Autodesk Inventor part; units mm, degrees
ref_plane "YZ Plane" through (0, 0, 0) normal (1, 0, 0) x (0, 1, 0)
ref_plane "XZ Plane" through (0, 0, 0) normal (0, 1, 0) x (-1, 0, 0)
ref_plane "XY Plane" through (0, 0, 0) normal (0, 0, 1) x (1, 0, 0)
sketch "スケッチ1" plane through (0, 0, 0) normal (1, 0, 0) x (0, 1, 0)
  line L0 (-670, 192.9198) -> (-670, 500)
  line L1 (-670, 500) -> (-350, 650)
  line L2 (-350, 650) -> (-90, 650)
  line L3 (0, 250) -> (0, 0)
  line L4 (-124.5856, 512.0252) -> (-145.1979, 512.0252)
  line L5 (-145.1979, 512.0252) -> (0, 250)
  line L6 (-90, 650) -> (-124.5856, 512.0252)
  line L7 (-249.1712, 52.2397) -> (-510, 192.9198)
  line L8 (-510, 192.9198) -> (-670, 192.9198)
  line L9 (0, 0) -> (-249.1712, 52.2397)
  dimension "d2" = 150
  dimension "d3" = 320
  dimension "d4" = 250
  dimension "d5" = 670
  dimension "d79" = 260
extrude "押し出し1" add sketch "スケッチ1" along normal blind 5
sketch "スケッチ8" plane through (5, 0, 0) normal (1, 0, 0) x (0, 0, -1)
  circle A0 centre (-570, -250) radius 7.5
  circle A1 centre (-288.2903, -224.7089) radius 7.5
  line L0 (0, 0) -> (-250, 0)
  line L1 (-570, -250) -> (-290.3837, -264.6541)
  line L2 (-290.3837, -264.6541) -> (-288.2903, -224.7089)
  line L3 (0, -804) -> (0, 134)
  dimension "d65" = 15
  dimension "d66" = 15
  dimension "d77" = 250
  dimension "d88" = 40
  dimension "d89" = 280
  dimension "d90" = 3
  dimension "d91" = 570
extrude "押し出し8" cut sketch "スケッチ8" against normal through all
sketch "スケッチ12" plane through (5, 0, 0) normal (1, 0, 0) x (0, 0, -1)
  circle A0 centre (-200, -95) radius 6.6799
  point P0 (0, 0)
  dimension "d84" = 200
  dimension "d85" = 95
extrude "押し出し11" cut sketch "スケッチ12" against normal through all
sketch "スケッチ13" plane through (5, 0, 0) normal (1, 0, 0) x (0, 0, -1)
  line L0 (0, -804) -> (0, 134)
  line L1 (130, 0) -> (-780, 0)
  line L2 (-80, 0) -> (-121.7476, -89.528)
  line L3 (-121.7476, -89.528) -> (-1.0516, -5.0157)
  line L4 (-52.2397, -249.1712) -> (0, 0)
  dimension "d95" = 80
  dimension "d96" = 115
  dimension "d97" = 30
extrude "押し出し12" cut sketch "スケッチ13" against normal through all
fillet "フィレット2" radius 3 6 edges at (2.5, -89.528, 121.7476) (2.5, -5.0157, 1.0516) (2.5, 0, 80) (2.5, -145.1979, 512.0252) (2.5, -124.5856, 512.0252) (2.5, -90, 650)
sketch "スケッチ14" plane through (5, 0, 0) normal (1, 0, 0) x (0, 0, -1)
  line L0 (-117.0159, -79.3808) -> (-81.9901, -4.2679)
  line L1 (-52.2397, -249.1712) -> (-2.608, -12.4393)
  line L2 (-7.2648, -9.3663) -> (-112.5762, -83.1061)
  line L3 (-81.9901, -4.2679) -> (-139.0675, -126.6706)
  line L4 (-139.0675, -126.6706) -> (-12.3616, -58.9618)
  line L5 (-52.2397, -249.1712) -> (-2.608, -12.4393)
  line L6 (-12.3616, -58.9618) -> (-2.608, -12.4393)
  line L7 (-2.608, -12.4393) -> (0, 0)
  line L8 (0, 0) -> (-81.9901, -4.2679)
extrude "押し出し13" cut sketch "スケッチ14" against normal through all
properties part number "end_plate" material "木材 (オーク)"
Geometry: final body of the model. Coordinates: model frame, mm. A direction names the side the tool comes from. Round coordinates to 2 decimals unless told otherwise and drop trailing zeros. Loops run counter-clockwise (first coordinate to the right, second up) from the corner with the lowest first, then second, coordinate; pieces in that order, holes last. Notation, with made-up numbers: (23.5, 79) - (47.5, 79) arc R22 ccw to (47.5, 106) - close; hole circle Ø6 at (86.25, 48.5). An arc over 180 degrees is marked (long way). Write each question's results on one line, items separated by ' | '. Start each with the question number.
1) Cut plane B-B on x = 2.65. Return loops of the section in (y, z).
2) Line query: probe 1 along Z at (x, y) = (3, -250); probe 2 along Y at (x, z) = (3.5, 570); probe 3 along Z at (x, y) = (4.65, -220.5). Output: solid intervals per line, ascending. Write a range as [from, to].
3) Cut plane D-D on z = 153.5. Return loops of the section in (x, y), then the cut area to 3 significant figures.
4) Access query for faces 1 (the face through (2.54, -93.29, 76.6)), 2 (the face through (2.465, -152.735, 32.021)), 3 (the face through (2.465, -72.364, 380.589)). Directions: +Z, -Z, +X, -X, +Y, -Y. A direction counts if a zero-diameter tool reaches every point of the face in a straight line with its end or side. Return the directions, or none.
5) Mould query, pull axis Y, two halves, no side actions, for faces 4 (the face through (2.535, -247.747, 562.846)), 5 (the face through (0, -340, 336)), 6 (the face through (2.465, -107.244, 581.207)). Classes: released by +Y, released by -Y, zero draft, split by the parting line, or undercut.
6) First-contact query: P1, Ø3, axis at x = 1, y = -177.5, coming from the -Z side; P2, Ø12, axis at y = -250, z = 570, coming from the +X side; P3, Ø1.5, axis at x = 3.5, y = -136, coming from the -Z side. Flat tips, straight axial feed; report the tip coordinate or a pass-through.
7) Cut plane C-C on y = -597. Return loops of the section in (x, z).
8) Cut plane A-A on z = 570. Return loops of the section in (x, y), then the cut area to 3 significant figures.
Verdict:
1) outline: (-670, 192.92) - (-510, 192.92) - (-249.17, 52.24) - (-58.96, 12.36) - (-126.67, 139.07) - (-79.38, 117.02) - (-4.27, 81.99) arc R3 ccw to (0, 84.71) - (0, 250) - (-142.73, 507.57) arc R3 cw to (-140.11, 512.03) - (-126.93, 512.03) arc R3 ccw to (-124.02, 514.3) - (-90.93, 646.27) arc R3 ccw to (-93.84, 650) - (-350, 650) - (-670, 500) - close; hole circle Ø15 at (-250, 570); hole circle Ø15 at (-224.71, 288.29); hole circle Ø13.36 at (-95, 200)
2) probe 1: z = [52.69, 562.5], [577.5, 650] | probe 2: y = [-520.67, -257.5], [-242.5, -110.05] | probe 3: z = [46.23, 282.08], [294.5, 650]
3) outline: (0, -436.91) - (5, -436.91) - (5, 0) - (0, 0) - close | area: 2,180 mm2
4) face 1: +X, -X | face 2: -Z, +X, -X, -Y | face 3: +X, -X, +Y
5) face 4: undercut | face 5: zero draft | face 6: released by +Y
6) P1: stops at z = 36.9 | P2: passes through | P3: stops at z = 28.36
7) outline: (0, 192.92) - (5, 192.92) - (5, 534.22) - (0, 534.22) - close
8) outline: (0, -520.67) - (5, -520.67) - (5, -257.5) - (0, -257.5) - close; (0, -242.5) - (5, -242.5) - (5, -110.05) - (0, -110.05) - close | area: 1,980 mm2
